```python
from build123d import *

# Parameters (mm, degrees)
F3_D     = 5
F3_DEPTH = 11.501
F4_SIZE  = 1


with BuildPart() as f1:
    # F0 (on Front) → F1 (revolve)
    with BuildSketch(Plane.XZ):
        Polygon((-15.895556457, 11.5), (-25, 5.125), (0, 5.125), (0, 11.5), align=None)
    revolve(axis=Axis((-30.6950435042, 0, 0), (1, 0, 0)))

    # F3 (through all, one way)
    with BuildSketch(Plane(origin=(0, 0, 0), x_dir=(1, 0, 0), z_dir=(0, 0, -1))):
        with Locations((-7.9477782285, 0)):
            Circle(F3_D / 2)
    extrude(amount=-F3_DEPTH, mode=Mode.SUBTRACT)

    # F4
    f4_edges = [f1.edges().sort_by_distance(p)[0] for p in [
        (0, 0, -11.5),
    ]]
    chamfer(f4_edges, length=F4_SIZE)


solid = f1.part
```
Source: CAD feature listing. Evaluate the final solid. Frame: model axes, mm. Round coordinates to 2 decimals unless told otherwise and drop trailing zeros. Write each loop counter-clockwise with the first axis right and the second up, starting at its lowest first coordinate (ties: lowest second). Pieces come first, ordered by that corner, then holes. Notation, with made-up numbers: M 83.5,84.5 L 106.5,84.5 A19 ccw 106.5,119.5 Z; hole C 19.5,67 d4. An arc over 180 degrees is marked long. Use CSV: the item, a comma, the result in double quotes. Start each with the question number.
Q1. Cut plane C-C on x = -14.5. Output: boundary loops of the cut face in (y, z) (3 decimals).
Q2. First-contact query: P1, Ø3, axis at x = -3.5, z = -7.5, coming from the +Y side; P2, Ø2, axis at x = -18, z = 3.5, coming from the +Y side; P3, Ø3, axis at x = -3.5, y = -4.5, coming from the +Z side; P4, Ø12, axis at x = -8, z = 1, coming from the -Y side. Flat tips, straight axial feed; report the tip coordinate or a pass-through.
Q3. Line query: line 1 (Y direction, x = -14.5, z = 0) (3 decimals); line 2 (Z direction, x = -9.5, y = 0) (3 decimals). Output: solid intervals per line, ascending. Write a range as from..to.
Q4. Cut plane A-A on y = 0. Output: boundary loops of the cut face in (x, z) (3 decimals), plus the area to 3 significant figures.
Q5. Pull-direction query (Y, two-part tool) for faces 1 (the face through (0, -2, -5)), 2 (the face through (-5.64, 0.96, 7.94)), 3 (the face through (-24.56, 4.82, 2.51)); classes: +Y half, -Y half, draft (parallel to the pull), parting line (faces both ways), or undercut.
Q6. Cut plane B-B on z = 0. Output: boundary loops of the cut face in (x, y) (3 decimals).
Q7. Cut plane D-D on x = -7.5. Output: boundary loops of the cut face in (y, z) (3 decimals).
Results found:
1,outline,"C 0,0 d23; hole C 0,0 d10.25"
2,P1,"y = 9.81"
2,P2,"y = 10.21"
2,P3,"z = 11.1"
2,P4,"y = -11.5"
3,line 1,"-11.5..-5.125, 5.125..11.5"
3,line 2,"-11.5..-5.125"
4,outline,"M -25,-5.125 L -15.896,-11.5 L -1,-11.5 L 0,-10.5 L 0,-5.125 Z; M -25,5.125 L -10.448,5.125 L -10.448,11.5 L -15.896,11.5 Z; M -5.448,5.125 L 0,5.125 L 0,10.5 L -1,11.5 L -5.448,11.5 Z"
4,area,"228 mm^2"
5,face 1,"draft"
5,face 2,"undercut"
5,face 3,"parting line"
6,outline,"M -25,-5.125 L -15.896,-11.5 L -1,-11.5 L 0,-10.5 L 0,-5.125 Z; M -25,5.125 L 0,5.125 L 0,10.5 L -1,11.5 L -15.896,11.5 Z"
7,outline,"M -2.46,4.496 L -2.46,11.234 A11.5 ccw long 2.46,11.234 L 2.46,4.496 A5.125 cw long Z"
